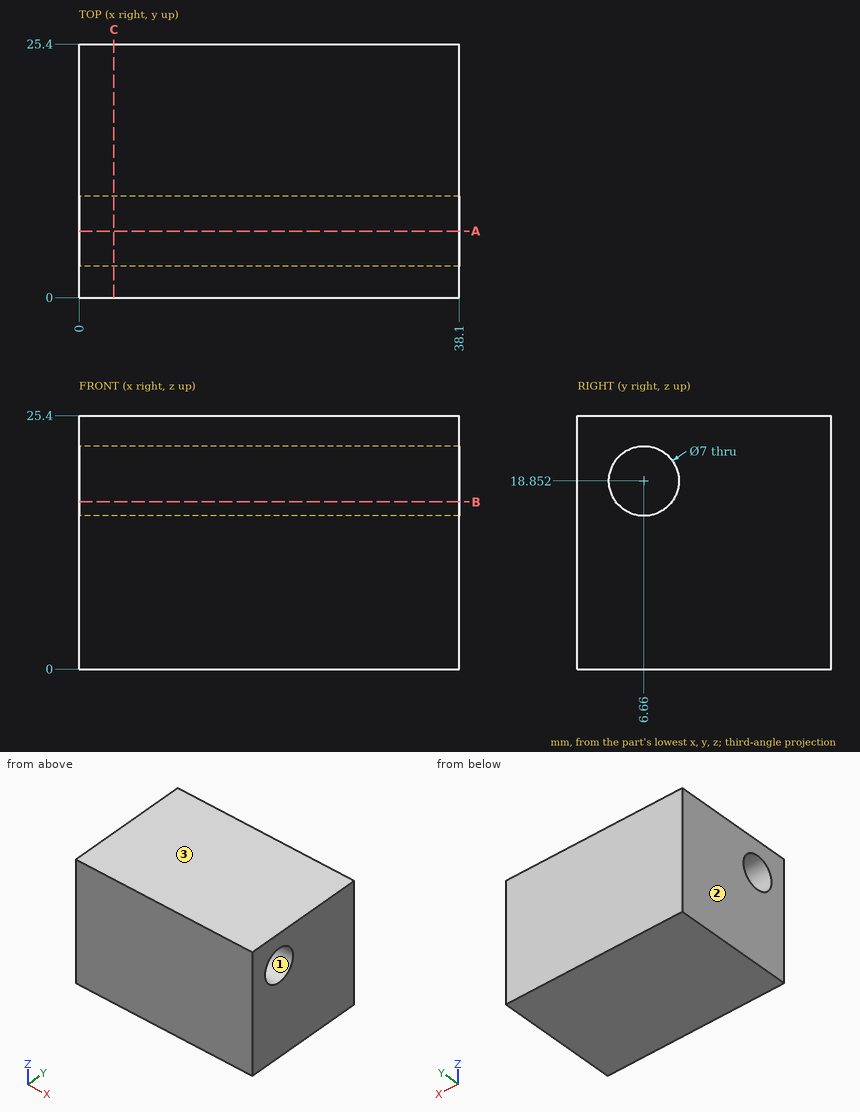
Geometry: see drawing. Coordinates: mm, zero at the bounding-box minimum. Round coordinates to 2 decimals unless told otherwise and drop trailing zeros. Loops run counter-clockwise (first coordinate to the right, second up) from the corner with the lowest first, then second, coordinate; pieces in that order, holes last. Notation, with made-up numbers: (79.25, -13) - (138.25, -13) arc R23 cw to (138.25, 0) - close; hole circle Ø5 at (4, -32). An arc over 180 degrees is marked (long way). One line per item, written item: value. Start each with the question number.
(1) Draft query along Z for the marked faces 1, 2 and 3. Return one class per face: +Z half, -Z half, draft (parallel to the pull), parting line (faces both ways), or undercut.
(2) Ray query, line 1 (Z direction, x = 19, y = 6.66); line 2 (Z direction, x = 27, y = 6.5); line 3 (Y direction, x = 36.5, z = 19). Return the intervals inside material, ascending. Write a range as [from, to].
(3) Section A-A, the plane y = 6.66. Return loops of the section in (x, z), plus the area to 3 significant figures.
(4) Section C-C, the plane x = 3.5. Return loops of the section in (y, z), plus the area to 3 significant figures.
(5) Section B-B, the plane z = 16.75. Return loops of the section in (x, y).
Results below:
1. face 1: undercut
1. face 2: draft
1. face 3: +Z half
2. line 1: [0, 15.35], [22.35, 25.4]
2. line 2: [0, 15.36], [22.35, 25.4]
2. line 3: [0, 3.16], [10.16, 25.4]
3. outline: (0, 0) - (38.1, 0) - (38.1, 15.35) - (0, 15.35) - close; (0, 22.35) - (38.1, 22.35) - (38.1, 25.4) - (0, 25.4) - close
3. area: 701 mm^2
4. outline: (0, 0) - (25.4, 0) - (25.4, 25.4) - (0, 25.4) - close; hole circle Ø7 at (6.66, 18.85)
4. area: 607 mm^2
5. outline: (0, 0) - (38.1, 0) - (38.1, 3.86) - (0, 3.86) - close; (0, 9.46) - (38.1, 9.46) - (38.1, 25.4) - (0, 25.4) - close
